Autodesk Inventor part; units mm, degrees
ref_plane "YZ Plane" through (0, 0, 0) normal (1, 0, 0) x (0, 1, 0)
ref_plane "XZ Plane" through (0, 0, 0) normal (0, 1, 0) x (-1, 0, 0)
ref_plane "XY Plane" through (0, 0, 0) normal (0, 0, 1) x (1, 0, 0)
sketch "Sketch1" plane through (0, 0, 0) normal (0, 1, 0) x (-1, 0, 0)
  line L0 (7.9375, 0) -> (23.8125, 0)
  line L1 (31.75, -7.9375) -> (31.75, -73.025)
  line L2 (23.8125, -80.9625) -> (7.9375, -80.9625)
  line L3 (0, -73.025) -> (0, -7.9375)
  arc A0 (31.75, -7.9375) -> (23.8125, 0) centre (23.8125, -7.9375) ccw
  arc A1 (23.8125, -80.9625) -> (31.75, -73.025) centre (23.8125, -73.025) ccw
  arc A2 (0, -73.025) -> (7.9375, -80.9625) centre (7.9375, -73.025) ccw
  arc A3 (7.9375, 0) -> (0, -7.9375) centre (7.9375, -7.9375) ccw
  point P0 (0, 0)
  point P1 (31.75, -80.9625)
  point P2 (31.75, 0)
  point P3 (0, -80.9625)
  dimension "d0" = 80.9625
  dimension "d1" = 31.75
  dimension "d2" = 7.9375
  dimension "d3" = 7.9375
  dimension "d4" = 7.9375
  dimension "d5" = 7.9375
extrude "Extrusion1" add sketch "Sketch1" along normal blind 12.446
sketch "Sketch2" plane through (0, 12.446, 0) normal (0, 1, 0) x (1, 0, 0)
  line L0 (-31.75, 73.025) -> (-31.75, 7.9375)
  line L1 (-31.75, 3.952) -> (-31.496, 3.952)
  line L2 (-23.8125, 0) -> (-7.9375, 0)
  line L3 (-15.875, 0) -> (-15.875, 0.254)
  line L4 (-7.9375, 80.9625) -> (-23.8125, 80.9625)
  line L5 (-15.875, 80.9625) -> (-15.875, 80.7085)
  line L6 (0, 7.9375) -> (0, 73.025)
  line L7 (0, 40.4812) -> (-0.254, 40.4812)
  line L8 (-23.5585, 0.254) -> (-8.1915, 0.254)
  line L9 (-0.254, 8.1915) -> (-0.254, 72.771)
  line L10 (-8.1915, 80.7085) -> (-23.5585, 80.7085)
  line L11 (-31.496, 72.771) -> (-31.496, 8.1915)
  arc A0 (-0.254, 72.771) -> (-8.1915, 80.7085) centre (-8.1915, 72.771) ccw
  arc A1 (-23.5585, 80.7085) -> (-31.496, 72.771) centre (-23.5585, 72.771) ccw
  arc A2 (-8.1915, 0.254) -> (-0.254, 8.1915) centre (-8.1915, 8.1915) ccw
  arc A3 (-31.496, 8.1915) -> (-23.5585, 0.254) centre (-23.5585, 8.1915) ccw
  point P0 (0, 0)
  dimension "d8" = 0.254
  dimension "d9" = 0.254
  dimension "d10" = 0.254
  dimension "d11" = 0.254
  dimension "d12" = 7.9375
extrude "Extrusion2" cut sketch "Sketch2" against normal blind 0.1016
sketch "Sketch3" plane through (-31.75, 0, -73.025) normal (-1, 0, 0) x (0, 0, 1)
  line L0 (65.0875, 0) -> (0, 0)
  line L1 (59.5609, 0) -> (59.5609, 5.08)
  line L2 (65.0875, 12.446) -> (65.0875, 6.604)
  line L3 (65.0875, 0) -> (65.0875, 12.446)
  line L4 (58.7672, 5.08) -> (54.0047, 5.08)
  line L5 (53.2109, 5.8737) -> (53.2109, 5.8737)
  line L6 (54.0047, 6.6675) -> (58.7672, 6.6675)
  line L7 (59.5609, 5.8737) -> (59.5609, 5.8737)
  arc A0 (54.0047, 6.6675) -> (53.2109, 5.8737) centre (54.0047, 5.8738) ccw
  arc A1 (53.2109, 5.8737) -> (54.0047, 5.08) centre (54.0047, 5.8737) ccw
  arc A2 (59.5609, 5.8737) -> (58.7672, 6.6675) centre (58.7672, 5.8738) ccw
  arc A3 (58.7672, 5.08) -> (59.5609, 5.8737) centre (58.7672, 5.8737) ccw
  point P0 (73.025, 0)
  point P1 (53.2109, 6.6675)
  point P2 (59.5609, 6.6675)
  dimension "d15" = 5.08
  dimension "d17" = 5.842
  dimension "d18" = 6.35
  dimension "d19" = 1.5875
  dimension "d20" = 0.7937
extrude "Extrusion3" cut sketch "Sketch3" against normal blind 0.0254
sketch "Sketch4" plane through (0, 0, 0) normal (0, -1, 0) x (1, 0, 0)
  line L0 (-23.5585, -0.254) -> (-8.1915, -0.254)
  line L1 (-0.254, -8.1915) -> (-0.254, -72.771)
  line L2 (-8.1915, -80.7085) -> (-23.5585, -80.7085)
  line L3 (-31.496, -72.771) -> (-31.496, -8.1915)
  arc A0 (-31.496, -72.771) -> (-23.5585, -80.7085) centre (-23.5585, -72.771) ccw
  arc A1 (-8.1915, -80.7085) -> (-0.254, -72.771) centre (-8.1915, -72.771) ccw
  arc A2 (-23.5585, -0.254) -> (-31.496, -8.1915) centre (-23.5585, -8.1915) ccw
  arc A3 (-0.254, -8.1915) -> (-8.1915, -0.254) centre (-8.1915, -8.1915) ccw
  point P0 (0, 0)
  dimension "d23" = 7.9375
  dimension "d24" = 7.9375
  dimension "d25" = 7.9375
  dimension "d26" = 7.9375
extrude "Extrusion4" add sketch "Sketch4" along normal blind 0.0508
properties part number "leapmotioncontroller"
Design review of the part built by this model. Coordinates are the model's own, in mm. Coordinates: 2 decimals unless noted, no trailing zeros. Order: outer loops, then holes, each group sorted by start corner. A loop starts at its lowest first (then second) coordinate and runs counter-clockwise, first axis right, second up. Notation, with made-up numbers: (40, 59) -> (53, 59) arc R18 cw to (53, 72) -> close; hole circle Ø3 at (-35.75, 44.5). An arc over 180 degrees is marked (long way). One line per item, written item: value. Start each with the question number.
Q1. Insertion check: pin 1 Ø3 at (y, z) = (4, -21) entering from +X; pin 2 Ø9.5 at (x, z) = (-20.5, -51) entering from +Y; pin 3 Ø0.5 at (y, z) = (6, -16.5) entering from -X. Each pin has a flat end and moves straight along its axis. Give the tip position at first contact, or say it passes through.
Q2. Take a section at C-C, the plane x = -30. State the section outline as (y, z) points.
Q3. For probe 1 along Y at (x, z) = (-20.5, -18); probe 2 along Z at (x, y) = (-6, 1.75); probe 3 along Z at (x, y) = (-25.5, 8.75), list the stretches that pass through material, from the lowest coordinate up.
Q4. Take a section at B-B, the plane x = -4.5. State the section outline as (y, z) points, then the cut area to 3 significant figures.
Values follow:
1. pin 1: stops at x = 0
1. pin 2: stops at y = 12.34
1. pin 3: stops at x = -31.72
2. outline: (-0.05, -77.41) -> (0, -77.41) -> (0, -78) -> (12.45, -78) -> (12.45, -77.41) -> (12.34, -77.41) -> (12.34, -3.55) -> (12.45, -3.55) -> (12.45, -2.97) -> (0, -2.97) -> (0, -3.55) -> (-0.05, -3.55) -> close
3. probe 1: y = -0.05 to 12.34
3. probe 2: z = -80.72 to -0.24
3. probe 3: z = -80.78 to -0.18
4. outline: (-0.05, -79.8) -> (0, -79.8) -> (0, -80.18) -> (12.45, -80.18) -> (12.45, -79.8) -> (12.34, -79.8) -> (12.34, -1.16) -> (12.45, -1.16) -> (12.45, -0.78) -> (0, -0.78) -> (0, -1.16) -> (-0.05, -1.16) -> close
4. area: 984 mm2
